Build history of the part. All positions in model axes, mm. Face numbers are marked on the shaded views. A direction names the side the tool comes from. Round coordinates to 2 decimals unless told otherwise and drop trailing zeros. Order: outer loops, then holes, each group sorted by start corner. A loop starts at its lowest first (then second) coordinate and runs counter-clockwise, first axis right, second up. Notation, with made-up numbers: (-24.5, 63.5) -> (-20.5, 63.5) arc R10 cw to (-20.5, 77.5) -> close; hole circle Ø8 at (20.25, 77). An arc over 180 degrees is marked (long way). Answer as a JSON object with one key per item and string values.
Autodesk Inventor part; units mm, degrees
ref_plane "YZ Plane" through (0, 0, 0) normal (1, 0, 0) x (0, 1, 0)
ref_plane "XZ Plane" through (0, 0, 0) normal (0, 1, 0) x (-1, 0, 0)
ref_plane "XY Plane" through (0, 0, 0) normal (0, 0, 1) x (1, 0, 0)
sketch "スケッチ1" plane through (0, 0, 0) normal (0, 0, 1) x (1, 0, 0)
  line L0 (-16, -16) -> (16, -16)
  line L1 (16, -16) -> (16, 16)
  line L2 (16, 16) -> (-16, 16)
  line L3 (-16, 16) -> (-16, -16)
  line L4 (-16, -16) -> (16, 16) construction
  line L5 (16, -16) -> (-16, 16) construction
  line L6 (-14.4, 14.4) -> (14.4, 14.4)
  line L7 (14.4, 14.4) -> (14.4, -14.4)
  line L8 (14.4, -14.4) -> (-14.4, -14.4)
  line L9 (-14.4, -14.4) -> (-14.4, 14.4)
  point P0 (0, 0)
  dimension "d0" = 32
  dimension "d1" = 32
  dimension "d2" = 1.6
extrude "押し出し1" add sketch "スケッチ1" along normal blind 95
sketch "スケッチ2" plane through (-16, 16, 0) normal (0, 1, 0) x (1, 0, 0)
  circle A0 centre (16, 0) radius 13.6
  dimension "d5" = 27.2
extrude "押し出し2" cut sketch "スケッチ2" against normal blind 32
sketch "スケッチ3" plane through (-16, 16, 95) normal (0, 1, 0) x (1, 0, 0)
  line L0 (32, 0) -> (0, 0)
  point P0 (16, 95)
  point P1 (16, 15)
  dimension "d16" = 80
hole "穴1" at (0, 16, 80) direction (0, -1, 0) diameter 10.5 end through all
sketch "スケッチ4" plane through (-16, 16, 95) normal (0, 1, 0) x (1, 0, 0)
  circle A0 centre (16, 15) radius 13.6
  point P0 (16, 95)
  dimension "d17" = 80
  dimension "d18" = 27.2
properties part number "軸受上用"
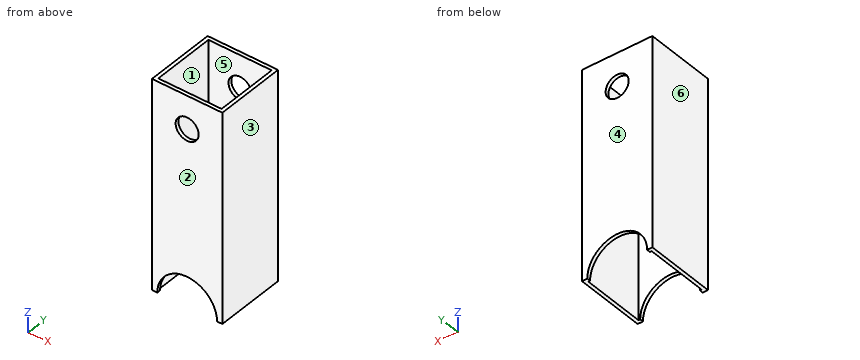
1) Cut at A-A, the plane x = 0. Give the cut face in (y, z), plus the area to 3 significant figures.
Checked values:
{"outline": "(-16, 13.6) -> (-14.4, 13.6) -> (-14.4, 74.75) -> (-16, 74.75) -> close; (-16, 85.25) -> (-14.4, 85.25) -> (-14.4, 95) -> (-16, 95) -> close; (14.4, 13.6) -> (16, 13.6) -> (16, 74.75) -> (14.4, 74.75) -> close; (14.4, 85.25) -> (16, 85.25) -> (16, 95) -> (14.4, 95) -> close", "area": "227 mm²"}
2) Cut at C-C, the plane y = 10. Give the cut face in (x, z), plus the area to 3 significant figures.
Checked values:
{"outline": "(-16, 0) -> (-14.4, 0) -> (-14.4, 95) -> (-16, 95) -> close; (14.4, 0) -> (16, 0) -> (16, 95) -> (14.4, 95) -> close", "area": "304 mm²"}
3) Which spindle directions (+Z, -Z, +X, -X, +Y, -Y) get a long thin tool onto all of the face, cutting with end or side? Do the marked faces 5 and 6. Say none if no direction does.
Checked values:
{"face 5": "+Z, -Z", "face 6": "+Z, -Z, -X, +Y, -Y"}
4) Probe L1, parallel to Y at x = -11, z = 61; L2, parallel to Z at x = 0, y = -15. List the from-to ranges inside material, lowest first. Write a range as from..to.
Checked values:
{"L1": "y = -16..-14.4, 14.4..16", "L2": "z = 13.6..74.75, 85.25..95"}
5) Cut at B-B, the plane z = 50.5. Give the cut face in (x, y).
Checked values:
{"outline": "(-16, -16) -> (16, -16) -> (16, 16) -> (-16, 16) -> close; hole (-14.4, -14.4) -> (14.4, -14.4) -> (14.4, 14.4) -> (-14.4, 14.4) -> close"}
6) Pull direction Y, two halves, no side cores. Call the marked faces 1, 2, 3 and 4: pulls with the +Y half, pulls with the -Y half, needs draft (parallel to the pull), parting line crosses it, or undercut.
Checked values:
{"face 1": "undercut", "face 2": "pulls with the -Y half", "face 3": "needs draft", "face 4": "pulls with the +Y half"}
7) Cut at D-D, the plane z = 80. Give the cut face in (x, y), plus the area to 3 significant figures.
Checked values:
{"outline": "(-16, -16) -> (-5.25, -16) -> (-5.25, -14.4) -> (-14.4, -14.4) -> (-14.4, 14.4) -> (-5.25, 14.4) -> (-5.25, 16) -> (-16, 16) -> close; (5.25, -16) -> (16, -16) -> (16, 16) -> (5.25, 16) -> (5.25, 14.4) -> (14.4, 14.4) -> (14.4, -14.4) -> (5.25, -14.4) -> close", "area": "161 mm²"}
